Study the drawing (mm; zero at the part's minimum x, y, z) and answer. A direction names the side the tool comes from. Give positions to 0.01 mm unless a question says otherwise; leave off trailing zeros. Loops run counter-clockwise (first coordinate to the right, second up) from the corner with the lowest first, then second, coordinate; pieces in that order, holes last. Notation, with made-up numbers: M 33,40.25 L 74,40.25 A22 ccw 74,71.25 Z; hole C 21.5,43.5 d11. An arc over 180 degrees is marked long. Use one line per item in the form item = value. Start each with the question number.
1. The part is cut by section A-A (x = 62). Write down the section's boundary in (y, z) (1 decimal).
2. Each of these flat-tipped pins is pushed along its axis until it touches: pin 1 Ø5 at (y, z) = (4.5, 54) entering from +X; pin 2 Ø4 at (x, z) = (50.5, 67.5) entering from +Y (1 decimal); pin 3 Ø21 at (x, z) = (48.2, 65) entering from -Y; pin 4 Ø12 at (x, z) = (65, 65) entering from +Y. Where does it stop, or does it pass through?
3. For the marked faces 1 and 2, determine the directions among +Z, -Z, +X, -X, +Y, -Y from which every point of the face is accessible in a straight line to the end or side of a thin tool.
4. The part is cut by section C-C (y = 13.5). Write down the section's boundary in (x, z) (1 decimal).
5. Straight lines are drawn through the part: line 1 (Z direction, x = 58.5, y = 9.5) (1 decimal); line 2 (X direction, y = 17, z = 65) (1 decimal); line 3 (X direction, y = 19.25, z = 60) (1 decimal). For each, find the intervals that lie inside material, in ascending order. Write a range as from..to.
6. The part is cut by section D-D (x = 45.5). Write down the section's boundary in (y, z) (1 decimal), and give its area (3 significant figures).
7. The part is cut by section B-B (z = 65). Write down the section's boundary in (x, y) (1 decimal).
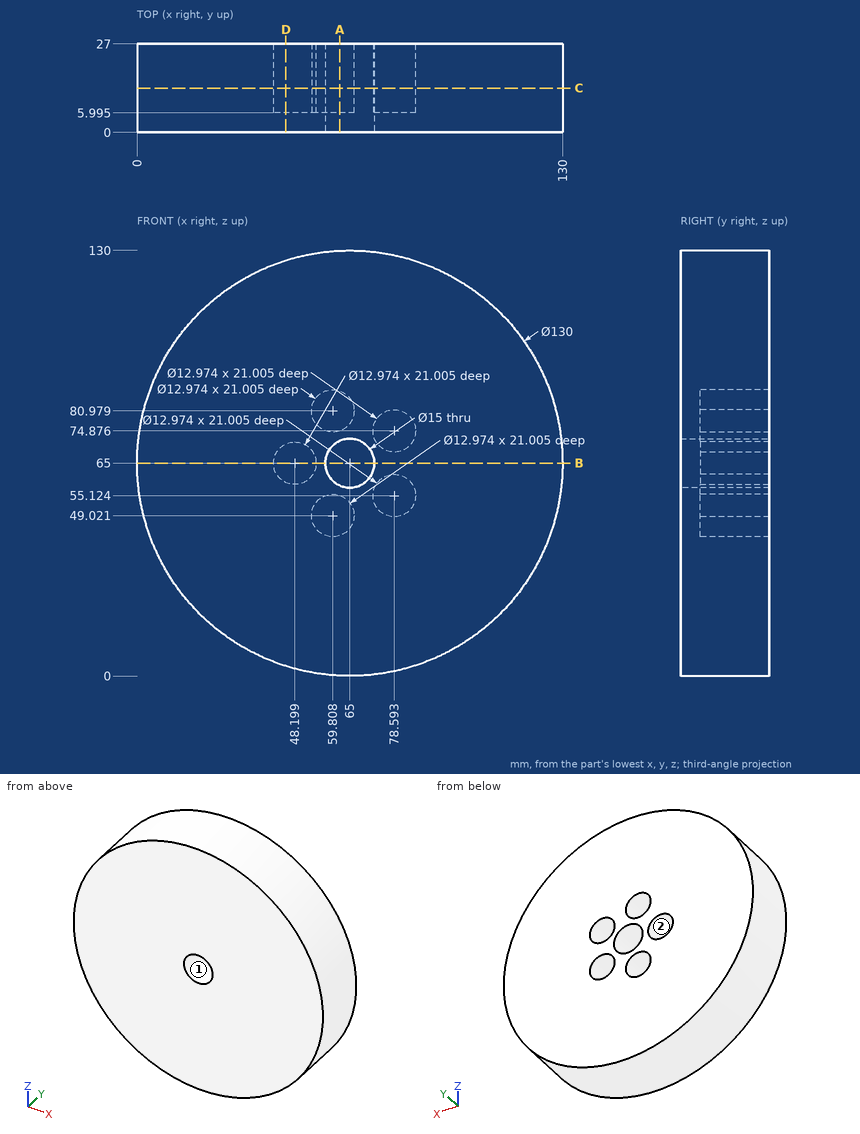
Derived:
q1.outline = M 0,0.1 L 27,0.1 L 27,42.9 L 6,42.9 L 6,55.1 L 27,55.1 L 27,58.1 L 0,58.1 Z; M 0,71.9 L 27,71.9 L 27,74.9 L 6,74.9 L 6,87.1 L 27,87.1 L 27,129.9 L 0,129.9 Z
q2.pin_1 = 129.44
q2.pin_2 = 6
q2.pin_3 = 0
q2.pin_4 = through
q3.face_1 = +Y, -Y
q3.face_2 = +Y
q4.outline = C 65,65 d130; hole C 48.2,65 d13; hole C 59.8,49 d13; hole C 59.8,81 d13; hole C 65,65 d15; hole C 78.6,55.1 d13; hole C 78.6,74.9 d13
q5.line_1 = 0.3..42.7, 55.4..61.3, 68.7..74.6, 87.3..129.7
q5.line_2 = 0..41.7, 54.7..57.5, 72.5..130
q5.line_3 = 0.2..44.1, 52.3..59.4, 70.6..74.3, 82.9..129.8
q6.outline = M 0,3 L 27,3 L 27,59.1 L 6,59.1 L 6,70.9 L 27,70.9 L 27,127 L 0,127 Z
q6.area = 3,100 mm2
q7.outline = M 0,0 L 57.5,0 L 57.5,27 L 54.7,27 L 54.7,6 L 41.7,6 L 41.7,27 L 0,27 Z; M 72.5,0 L 130,0 L 130,27 L 72.5,27 Z
